from build123d import *

# Parameters (mm, degrees)
RITNING_1_W          = 250
RITNING_1_H          = 9.8
KUGGST_NGS_MNE_DEPTH = 10
KUGGLUCKA_DEPTH      = 10
LPATTERN_COUNT       = 80
LPATTERN_PITCH       = 3.14159265
CUT_EXTRUDE1_DEPTH   = 10


with BuildPart() as part:
    # Ritning 1 → Kuggstångsämne (new body)
    with BuildSketch(Plane.XY):
        with Locations((0.9, 0)):
            Rectangle(RITNING_1_W, RITNING_1_H)
    extrude(amount=KUGGST_NGS_MNE_DEPTH)

    # Ritning 2 → Kugglucka (cut)
    with BuildSketch(Plane.XY.offset(10)):
        with BuildLine():
            Line((-124.438289352, 2.65), (-123.761710648, 2.65))
            Line((-123.761710648, 2.65), (-122.942777621, 4.9))
            Line((-122.942777621, 4.9), (-124.1, 6.057222379))
            Line((-124.1, 6.057222379), (-125.257222379, 4.9))
            add(Edge.make_bspline(
                [(-125.257222379, 4.9), (-124.984244704, 4.15), (-124.711267028, 3.4), (-124.438289352, 2.65)],
                knots=[0, 0, 0, 0, 1, 1, 1, 1], degree=3))
        make_face()
    kugglucka = extrude(amount=-KUGGLUCKA_DEPTH, mode=Mode.SUBTRACT)

    # LPattern: Kugglucka ×80
    with Locations(*[(i * LPATTERN_PITCH, 0, 0) for i in range(1, LPATTERN_COUNT)]):
        add(kugglucka, mode=Mode.SUBTRACT)

    # Sketch1 → Cut-Extrude1 (cut)
    with BuildSketch(Plane.XY.offset(10)):
        Polygon((-24.1, -4.9), (-24.1, 34.404726266), (165.055883849, 34.404726266), (170.123246632, -36.805056005), (-46.973243137, -44.806155137), align=None)
    extrude(amount=-CUT_EXTRUDE1_DEPTH, mode=Mode.SUBTRACT)


solid = part.part
Could you check a few things on this model? Use its own coordinates, in mm. A direction names the side the tool comes from. Give positions to 0.01 mm unless a question says otherwise; leave off trailing zeros. Answer as CSV lines item,"result". Start each with the question number.
(1) Please list where this line runs through material, in increasing order: line 1 (Y direction, x = -77, z = 5.25).
(2) I'm going to push a flat-ended pin straight in: pin 1 Ø0.5 at (x, z) = (-111.5, 7) entering from +Y. Where does the tip first touch, or does it pass through?
(3) If we mould it in two halves opening along X, with no side actions, what happens to faces 1 (the face through (-51.1, 3.76, 5.07)), 2 (the face through (-24.1, -1, 5)), 3 (the face through (-75, -4.9, 5)), 4 (the face through (-91.94, 3.76, 5.07))? For each: +X half, -X half, draft (parallel to the pull), parting line (faces both ways), or undercut.
(4) Which directions (+Z, -Z, +X, -X, +Y, -Y) give clear straight access to the entire face, cutting with the end or side of a thin tool? Please do faces 5 (the face through (-57.385, 3.759, 5.07)), 6 (the face through (-75, -1, 0)).
Answer list:
1,line 1,"-4.9 to 2.65"
2,pin 1,"y = 2.65"
3,face 1,"undercut"
3,face 2,"+X half"
3,face 3,"draft"
3,face 4,"undercut"
4,face 5,"+Z, -Z, +Y"
4,face 6,"-Z, +X, -X, +Y, -Y"
